The drawing under review shows one solid part. Ordinate dimensions are in mm from its lowest x, y, z. A direction names the side the tool comes from. Coordinates: 2 decimals unless noted, no trailing zeros. Loops run counter-clockwise (first coordinate to the right, second up) from the corner with the lowest first, then second, coordinate; pieces in that order, holes last.
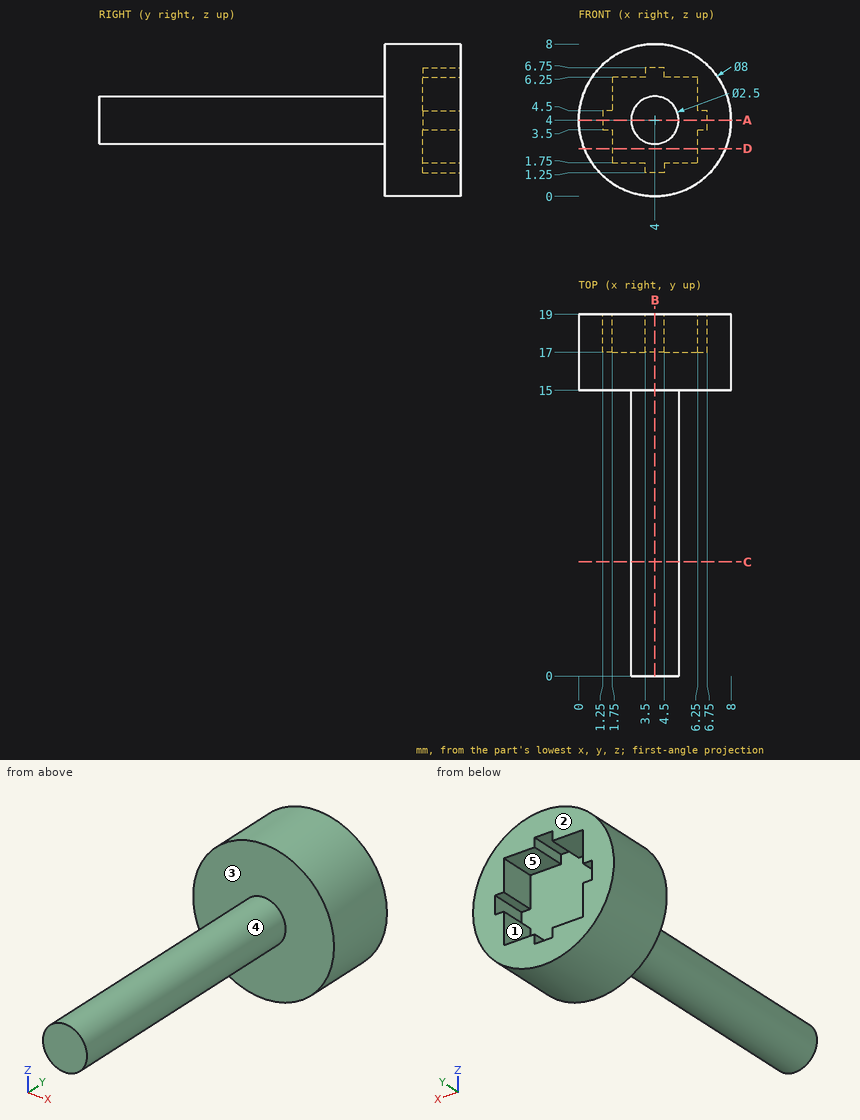
Q1. Clearance check with flat-ended pins moving along their axes: pin 1 Ø1.9 at (y, z) = (18.5, 5.5) entering from +X; pin 2 Ø1.5 at (y, z) = (13, 4) entering from +X; pin 3 Ø0.5 at (y, z) = (18, 5.5) entering from -X. State where each tip first meets the part, or that it passes through.
Q2. For line 1 (Y direction, x = 0.75, z = 2.5); line 2 (Y direction, x = 3.5, z = 6); line 3 (Z direction, x = 4, y = 13), list the stretches that pass through material, from the lowest coordinate up.
Q3. Machinability: for the marked faces 1 and 2, which of the approach directions +Z, -Z, +X, -X, +Y, -Y give a long, thin tool a straight path to every point of the face, cutting with its end or side? Answer none if there is none.
Q4. Take a section at C-C, the plane y = 6. Write out the cut boundary in (x, z).
Q5. Take a section at B-B, the plane x = 4. Write out the cut boundary in (y, z), then the cut area to 3 significant figures.
Q6. The part is to be moulded in two halves that separate along X. For the marked faces 3, 4 and 5, say which applies: pulls with the +X half, pulls with the -X half, needs draft (parallel to the pull), parting line crosses it, or undercut.
Q7. Take a section at A-A, the plane z = 4. Write out the cut boundary in (x, y).
Q8. Take a section at D-D, the plane z = 2.5. Write out the cut boundary in (x, y), then the cut area to 3 significant figures.
Entries:
1. pin 1: stops at x = 7.96
1. pin 2: stops at x = 5.25
1. pin 3: stops at x = 0.2
2. line 1: y = 15 to 19
2. line 2: y = 15 to 17
2. line 3: z = 2.75 to 5.25
3. face 1: +Y
3. face 2: +Z, -Z, +X, -X, +Y
4. outline: circle Ø2.5 at (4, 4)
5. outline: (0, 2.75) - (15, 2.75) - (15, 0) - (19, 0) - (19, 1.25) - (17, 1.25) - (17, 6.75) - (19, 6.75) - (19, 8) - (15, 8) - (15, 5.25) - (0, 5.25) - close
5. area: 58.5 mm2
6. face 3: needs draft
6. face 4: parting line crosses it
6. face 5: undercut
7. outline: (0, 15) - (2.75, 15) - (2.75, 0) - (5.25, 0) - (5.25, 15) - (8, 15) - (8, 19) - (6.75, 19) - (6.75, 17) - (1.25, 17) - (1.25, 19) - (0, 19) - close
8. outline: (0.29, 15) - (7.71, 15) - (7.71, 19) - (6.25, 19) - (6.25, 17) - (1.75, 17) - (1.75, 19) - (0.29, 19) - close
8. area: 20.7 mm2
